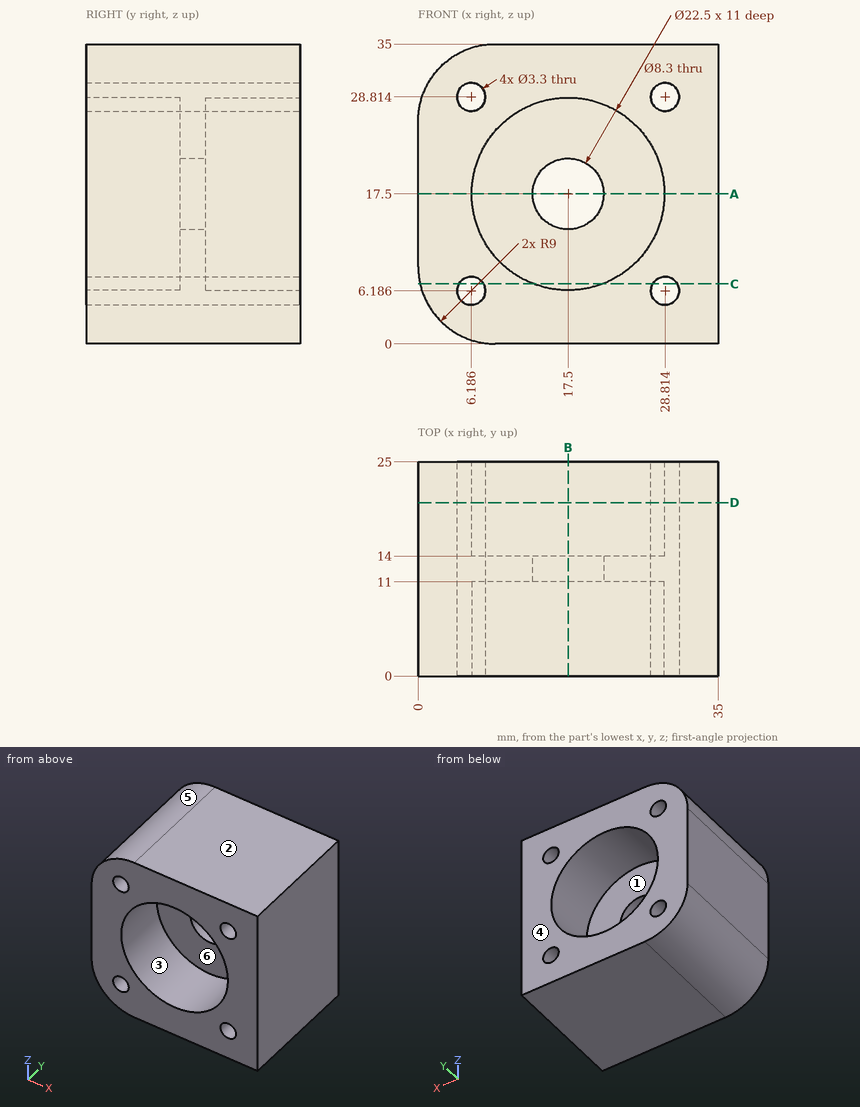
Geometry check sheet. Reference: drawing and pictorial views, mm from the part's lowest x, y, z. A direction names the side the tool comes from. Coordinates: 2 decimals unless noted, no trailing zeros. Loops run counter-clockwise (first coordinate to the right, second up) from the corner with the lowest first, then second, coordinate; pieces in that order, holes last. Notation, with made-up numbers: (-23, 44.5) -> (13, 44.5) arc R27 ccw to (13, 64.5) -> close; hole circle Ø7 at (-4.75, 52). An arc over 180 degrees is marked (long way). Put each result on its own line as item: value.
1) Cross-section at C-C on z = 7. Record the boundary of the cut face in (x, y) (1 decimal).
Result set:
outline: (0.2, 0) -> (4.8, 0) -> (4.8, 25) -> (0.2, 25) -> close; (7.6, 0) -> (13.5, 0) -> (13.5, 11) -> (21.5, 11) -> (21.5, 0) -> (27.4, 0) -> (27.4, 25) -> (21.5, 25) -> (21.5, 14) -> (13.5, 14) -> (13.5, 25) -> (7.6, 25) -> close; (30.2, 0) -> (35, 0) -> (35, 25) -> (30.2, 25) -> close
2) Cross-section at B-B on x = 17.5. Record the boundary of the cut face in (y, z).
Result set:
outline: (0, 0) -> (25, 0) -> (25, 6.25) -> (14, 6.25) -> (14, 13.35) -> (11, 13.35) -> (11, 6.25) -> (0, 6.25) -> close; (0, 28.75) -> (11, 28.75) -> (11, 21.65) -> (14, 21.65) -> (14, 28.75) -> (25, 28.75) -> (25, 35) -> (0, 35) -> close
3) Gauge pin test, flat ends, axial feed: pin 1 Ø4 at (y, z) = (18.5, 25) entering from -X; pin 2 Ø13.5 at (x, z) = (17.5, 17.5) entering from +Y; pin 3 Ø1 at (x, z) = (25, 18) entering from -Y; pin 4 Ø1.5 at (x, y) = (7, 18) entering from -Z. Record the tip position at first contact, or that the pin passes through.
Result set:
pin 1: stops at x = 0
pin 2: stops at y = 14
pin 3: stops at y = 11
pin 4: stops at z = 0.09
4) Thickness scan on line 1 (Z direction, x = 17.5, y = 3.5); line 2 (Z direction, x = 17.5, y = 12.7); line 3 (X direction, y = 4.5, z = 29.5) (1 decimal). Record the ranges inside material, lowest first.
Result set:
line 1: z = 0 to 6.25, 28.75 to 35
line 2: z = 0 to 13.35, 21.65 to 35
line 3: x = 0.7 to 4.7, 7.7 to 27.3, 30.3 to 35
5) Cross-section at D-D on y = 20.25. Record the boundary of the cut face in (x, z).
Result set:
outline: (0, 9) arc R9 ccw to (9, 0) -> (35, 0) -> (35, 35) -> (9, 35) arc R9 ccw to (0, 26) -> close; hole circle Ø3.3 at (6.19, 6.19); hole circle Ø3.3 at (6.19, 28.81); hole circle Ø22.5 at (17.5, 17.5); hole circle Ø3.3 at (28.81, 6.19); hole circle Ø3.3 at (28.81, 28.81)
6) Cross-section at A-A on z = 17.5. Record the boundary of the cut face in (x, y), plus the area to 3 significant figures.
Result set:
outline: (0, 0) -> (6.25, 0) -> (6.25, 11) -> (13.35, 11) -> (13.35, 14) -> (6.25, 14) -> (6.25, 25) -> (0, 25) -> close; (21.65, 11) -> (28.75, 11) -> (28.75, 0) -> (35, 0) -> (35, 25) -> (28.75, 25) -> (28.75, 14) -> (21.65, 14) -> close
area: 355 mm^2
7) Release check for a two-part mould opening along X. For the marked faces 4, 5 and 6 record: released by +X, released by -X, zero draft, split by the parting line, or undercut.
Result set:
face 4: zero draft
face 5: released by -X
face 6: undercut
8) Tool access check on the marked faces 1, 2 and 3. Record the directions out of +Z, -Z, +X, -X, +Y, -Y that give a thin tool (end or side, any length) a straight path to the whole face; none if there is none.
Result set:
face 1: +Y
face 2: +Z, +X, -X, +Y, -Y
face 3: -Y
